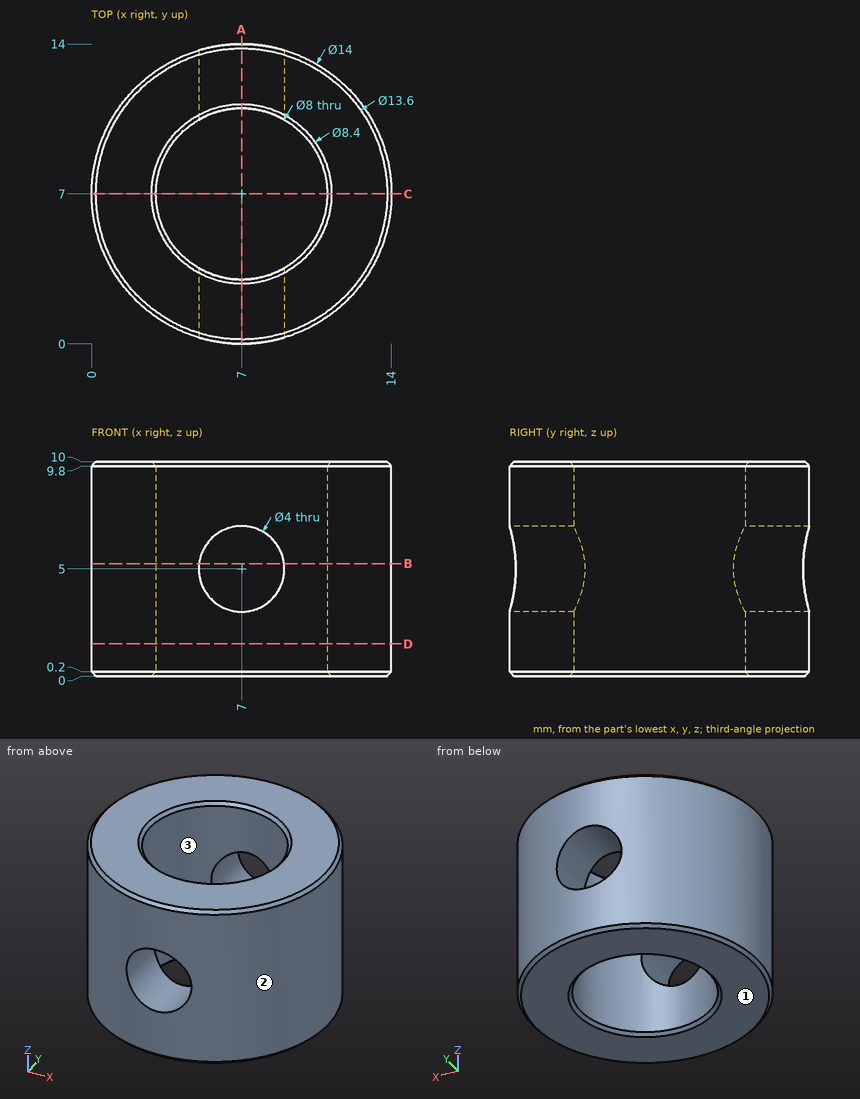
Drawing for the job (mm, zero at the part's lowest x, y, z). Give positions to 0.01 mm unless a question says otherwise; leave off trailing zeros. Write each loop counter-clockwise with the first axis right and the second up, starting at its lowest first coordinate (ties: lowest second). Pieces come first, ordered by that corner, then holes. Notation, with made-up numbers: (42.25, 83.5) - (76.25, 83.5) arc R15 ccw to (76.25, 96.5) - close; hole circle Ø7 at (83, 46). An arc over 180 degrees is marked (long way). Answer as CSV lines item,"result".
Q1. Band-saw the part on B-B (z = 5.25). Give the cut face in (x, y).
Result set:
outline,"(5.02, 0.29) - (5.02, 3.53) arc R4 cw to (5.02, 10.47) - (5.02, 13.71) arc R7 ccw to start; (8.98, 0.29) arc R7 ccw to (8.98, 13.71) - (8.98, 10.47) arc R4 cw to (8.98, 3.53) - close"
Q2. Pull direction X, two halves, no side cores. Call the marked faces 1, 2 and 3: released by +X, released by -X, zero draft, split by the parting line, or undercut.
Result set:
face 1,"zero draft"
face 2,"split by the parting line"
face 3,"undercut"
Q3. Band-saw the part on D-D (z = 1.5). Give the cut face in (x, y), and give its area (3 significant figures).
Result set:
outline,"circle Ø14 at (7, 7); hole circle Ø8 at (7, 7)"
area,"104 mm²"
Q4. Band-saw the part on C-C (y = 7). Give the cut face in (x, z).
Result set:
outline,"(0, 0.2) - (0.2, 0) - (2.8, 0) - (3, 0.2) - (3, 9.8) - (2.8, 10) - (0.2, 10) - (0, 9.8) - close; (11, 0.2) - (11.2, 0) - (13.8, 0) - (14, 0.2) - (14, 9.8) - (13.8, 10) - (11.2, 10) - (11, 9.8) - close"
Q5. Flat gauge pins, fed straight in: pin 1 Ø6 at (x, z) = (3.5, 1.5) entering from -Y; pin 2 Ø4 at (y, z) = (6.5, 5.5) entering from +X; pin 3 Ø1.5 at (x, z) = (2, 1.5) entering from +Y; pin 4 Ø7 at (x, y) = (7, 7) entering from +Z. Where does each tip first touch, or does it go through?
Result set:
pin 1,"y = 0.02"
pin 2,"x = 14"
pin 3,"y = 12.56"
pin 4,"through"
Q6. Band-saw the part on A-A (x = 7). Give the cut face in (y, z).
Result set:
outline,"(0, 0.2) - (0.2, 0) - (2.8, 0) - (3, 0.2) - (3, 3) - (0, 3) - close; (0, 7) - (3, 7) - (3, 9.8) - (2.8, 10) - (0.2, 10) - (0, 9.8) - close; (11, 0.2) - (11.2, 0) - (13.8, 0) - (14, 0.2) - (14, 3) - (11, 3) - close; (11, 7) - (14, 7) - (14, 9.8) - (13.8, 10) - (11.2, 10) - (11, 9.8) - close"
Q7. Drill centre lines: line 1 (Y direction, x = 7, z = 7.25); line 2 (Z direction, x = 7, y = 11.8); line 3 (Y direction, x = 4, z = 9.5). Where is each one in solid material? Low to high. Write a range as from..to.
Result set:
line 1,"0..3, 11..14"
line 2,"0..3, 7..10"
line 3,"0.68..4.35, 9.65..13.32"
